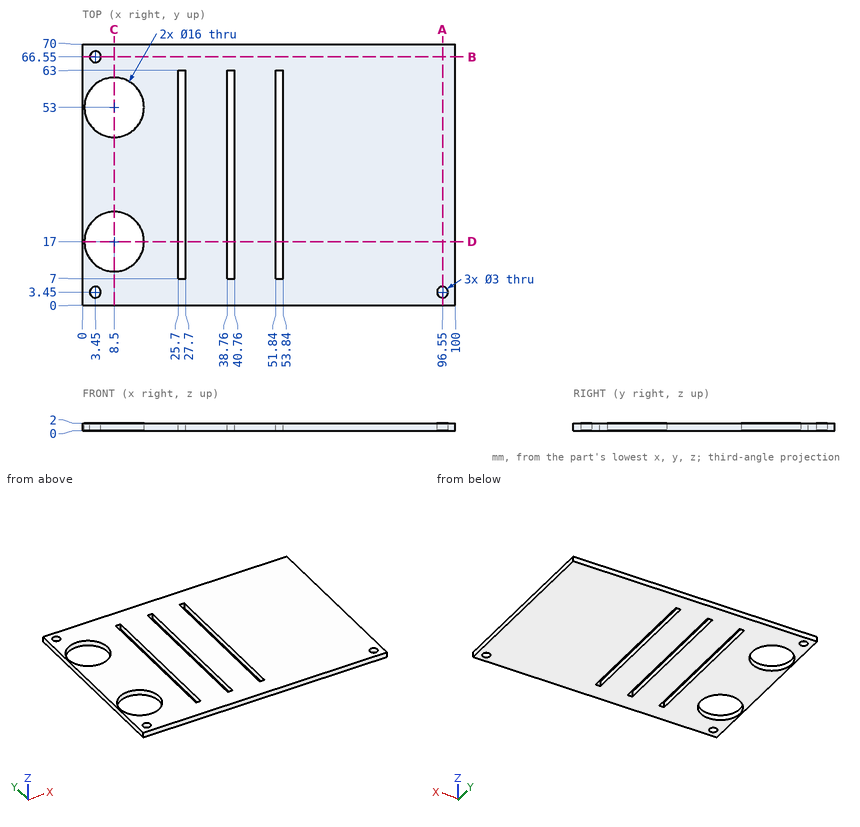
Geometry check sheet. Reference: drawing and pictorial views, mm from the part's lowest x, y, z. Round coordinates to 2 decimals unless told otherwise and drop trailing zeros. Loops run counter-clockwise (first coordinate to the right, second up) from the corner with the lowest first, then second, coordinate; pieces in that order, holes last. Notation, with made-up numbers: (0, 85.5) - (6, 85.5) arc R18 cw to (6, 108.5) - close; hole circle Ø7 at (84.25, 62.5). An arc over 180 degrees is marked (long way). Answer as CSV lines item,"result".
(1) Cross-section at B-B, the plane y = 66.55. Enter the section's corners in (x, z).
Output values:
outline,"(0, 0) - (1.95, 0) - (1.95, 2) - (0, 2) - close; (4.95, 0) - (100, 0) - (100, 2) - (4.95, 2) - close"
(2) Material ranges on line 1 along X through (y, z) = (28.5, 0.5); line 2 along Y through (x, z) = (8.5, 0.7); line 3 along Y through (x, z) = (3.45, 0.75), recorded low to high.
Output values:
line 1,"x = 0 to 25.7, 27.7 to 38.76, 40.76 to 51.84, 53.84 to 100"
line 2,"y = 0 to 9, 25 to 45, 61 to 70"
line 3,"y = 0 to 1.95, 4.95 to 10.8, 23.2 to 46.8, 59.2 to 65.05, 68.05 to 70"
(3) Cross-section at C-C, the plane x = 8.5. Enter the section's corners in (y, z), and give its area (3 significant figures).
Output values:
outline,"(0, 0) - (9, 0) - (9, 2) - (0, 2) - close; (25, 0) - (45, 0) - (45, 2) - (25, 2) - close; (61, 0) - (70, 0) - (70, 2) - (61, 2) - close"
area,"76.0 mm²"
(4) Cross-section at D-D, the plane y = 17. Enter the section's corners in (x, z).
Output values:
outline,"(0, 0) - (0.5, 0) - (0.5, 2) - (0, 2) - close; (16.5, 0) - (25.7, 0) - (25.7, 2) - (16.5, 2) - close; (27.7, 0) - (38.76, 0) - (38.76, 2) - (27.7, 2) - close; (40.76, 0) - (51.84, 0) - (51.84, 2) - (40.76, 2) - close; (53.84, 0) - (100, 0) - (100, 2) - (53.84, 2) - close"
(5) Cross-section at A-A, the plane x = 96.55. Enter the section's corners in (y, z), and give its area (3 significant figures).
Output values:
outline,"(0, 0) - (1.95, 0) - (1.95, 2) - (0, 2) - close; (4.95, 0) - (70, 0) - (70, 2) - (4.95, 2) - close"
area,"134 mm²"
